Input: part model. Units: mm. Frame: model coordinates. A direction names the side the tool comes from. Coordinates: 2 decimals unless noted, no trailing zeros. Order: outer loops, then holes, each group sorted by start corner. A loop starts at its lowest first (then second) coordinate and runs counter-clockwise, first axis right, second up. Notation, with made-up numbers: (-0.5, -8.5) - (50.5, -8.5) arc R31 cw to (50.5, 26.5) - close; hole circle Ø2 at (18, 39.25). An arc over 180 degrees is marked (long way). Answer as CSV lines item,"result". Start each with the question number.
Item 1: Section A-A (x = 0). Output: boundary loops of the cut face in (y, z) (3 decimals), and give its area (3 significant figures).
Item 2: Material intervals for line 1 along Y through (x, z) = (0, 22.55) (3 decimals); line 2 along X through (y, z) = (10.25, 22); line 3 along Z through (x, y) = (-28, 3.25), sorted ascending.
Item 3: Section B-B (y = 13.5). Output: boundary loops of the cut face in (x, z).
Item 4: Section D-D (z = -11.5). Output: boundary loops of the cut face in (x, y), and give its area (3 significant figures).
Item 5: Section C-C (x = 7). Output: boundary loops of the cut face in (y, z).
Item 6: First-contact query: pin 1 (3.5 mm diameter, centred on x = 0, y = 7.5, fed in from +Z); pin 2 (6 mm diameter, centred on x = -24, z = -12.5, fed in from -Y); pin 3 (7.5 mm diameter, centred on y = 9.5, z = -7, fed in from -X); pin 4 (8 mm diameter, centred on y = 7, z = 9, fed in from -X). Flat tips, straight axial feed; report the tip coordinate or a pass-through.
Item 7: Draft query along X for faces 4 (the flat face through (22, 8, 1)), 5 (the cylindrical face through (-26.537, 6.686, 22.535)), 6 (the flat face through (-32.2, 7.4, 17)). Return one class per face: +X half, -X half, draft (parallel to the pull), parting line (faces both ways), or undercut.
Item 8: Access query for faces 1 (the flat face through (0, 4, 18)), 2 (the flat face through (-26.9, 5.8, 20)), 3 (the flat face through (-1, 0, 17)). Directions: +Z, -Z, +X, -X, +Y, -Y. A direction counts if a zero-diameter tool reaches every point of the face in a straight line with its end or side. Return the directions, or none.
from build123d import *

# Parameters (mm, degrees)
CROQUIS1_R              = 15
SALIENTE_EXTRUIR1_DEPTH = 15
CORTAR_EXTRUIR1_REACH   = 62.49
CROQUIS2_R              = 2.125
CORTAR_EXTRUIR2_DEPTH   = 3
CUT_EXTRUDE1_DEPTH      = 46.552167984
CUT_EXTRUDE2_REACH      = 66.49
CUT_EXTRUDE2_END_RADIUS = 15
CUT_EXTRUDE2_START      = -4
CUT_EXTRUDE3_START      = -39
CUT_EXTRUDE3_DEPTH      = 3
BOSS_EXTRUDE3_START     = -15
BOSS_EXTRUDE3_DEPTH     = 15
CUT_EXTRUDE4_START      = -20
SKETCH4_R               = 1.625
CUT_EXTRUDE4_DEPTH      = 41.489668539


with BuildPart() as part:
    # Croquis1 → Saliente-Extruir1 (new body)
    with BuildSketch(Plane(origin=(0, 0, 0), x_dir=(1, 0, 0), z_dir=(0, 1, 0))):
        with BuildLine():
            Line((-35, -17), (-35, -25))
            Line((-35, -25), (35, -25))
            Line((35, -25), (35, -17))
            Line((35, -17), (25, -17))
            Line((25, -17), (22, 0))
            ThreePointArc((22, 0), (0, 22), (-22, 0))
            Line((-22, 0), (-25, -17))
            Line((-25, -17), (-35, -17))
        make_face()
        with Locations(Location((0, 0, 0), (0, 0, 270))):
            Circle(CROQUIS1_R, mode=Mode.SUBTRACT)
    extrude(amount=SALIENTE_EXTRUIR1_DEPTH)

    # Croquis2 → Cortar-Extruir1 (cut, up to next)
    with BuildSketch(Plane.XY.offset(25), mode=Mode.PRIVATE) as cortar_extruir1_sk1:
        with Locations((-28.5, 7.5)):
            Circle(CROQUIS2_R)
    cortar_extruir1_tool1 = extrude(cortar_extruir1_sk1.sketch, amount=-CORTAR_EXTRUIR1_REACH, mode=Mode.PRIVATE) & part.part
    # Croquis2 → Cortar-Extruir1 (cut, up to next)
    with BuildSketch(Plane.XY.offset(25), mode=Mode.PRIVATE) as cortar_extruir1_sk2:
        with Locations((28.5, 7.5)):
            Circle(CROQUIS2_R)
    cortar_extruir1_tool2 = extrude(cortar_extruir1_sk2.sketch, amount=-CORTAR_EXTRUIR1_REACH, mode=Mode.PRIVATE) & part.part
    # Croquis2 → Cortar-Extruir1 (cut, up to next)
    with BuildSketch(Plane.XY.offset(25), mode=Mode.PRIVATE) as cortar_extruir1_sk3:
        with Locations((0, 7.5)):
            Circle(CROQUIS2_R)
    cortar_extruir1_tool3 = extrude(cortar_extruir1_sk3.sketch, amount=-CORTAR_EXTRUIR1_REACH, mode=Mode.PRIVATE) & part.part
    add(cortar_extruir1_tool1.solids().sort_by_distance((-28.5, 7.5, 25))[0], mode=Mode.SUBTRACT)
    add(cortar_extruir1_tool2.solids().sort_by_distance((28.5, 7.5, 25))[0], mode=Mode.SUBTRACT)
    add(cortar_extruir1_tool3.solids().sort_by_distance((0, 7.5, 25))[0], mode=Mode.SUBTRACT)

    # Croquis3 → Cortar-Extruir2 (cut)
    with BuildSketch(Plane(origin=(0, 0, 17), x_dir=(-1, 0, 0), z_dir=(0, 0, -1))):
        Polygon((25, 5.479274058), (28.5, 3.458548116), (32, 5.479274058), (32, 9.520725942), (28.5, 11.541451884), (25, 9.520725942), align=None)
        Polygon((-25, 5.479274058), (-25, 9.520725942), (-28.5, 11.541451884), (-32, 9.520725942), (-32, 5.479274058), (-28.5, 3.458548116), align=None)
    extrude(amount=-CORTAR_EXTRUIR2_DEPTH, mode=Mode.SUBTRACT)

    # Sketch1 → Cut-Extrude1 (cut, through all)
    with BuildSketch(Plane(origin=(0, 15, 0), x_dir=(1, 0, 0), z_dir=(0, 1, 0))):
        Polygon((22, -25), (22, -20), (17, -25), align=None)
        Polygon((22, 0), (22, -20), (22, -25), (35, -25), (35, -17), (25, -17), align=None)
    extrude(amount=-CUT_EXTRUDE1_DEPTH, mode=Mode.SUBTRACT)

    # Cut-Extrude2: up to this cylinder (the profile starts outside it)
    cut_extrude2_end = Plane(origin=(0, 7.5, 0), z_dir=(0, -1, 0)) * Cylinder(CUT_EXTRUDE2_END_RADIUS, 163.98, mode=Mode.PRIVATE)
    # Sketch2 → Cut-Extrude2 (cut, up to the surface)
    with BuildSketch(Plane.XY.offset(25).offset(CUT_EXTRUDE2_START), mode=Mode.PRIVATE) as cut_extrude2_sk1:
        Polygon((2.020725942, 4), (4.041451884, 7.5), (2.020725942, 11), (-2.020725942, 11), (-4.041451884, 7.5), (-2.020725942, 4), align=None)
    cut_extrude2_tool1 = extrude(cut_extrude2_sk1.sketch, amount=-CUT_EXTRUDE2_REACH, mode=Mode.PRIVATE) - cut_extrude2_end
    add(cut_extrude2_tool1.solids().sort_by_distance((0, 7.5, 21))[0], mode=Mode.SUBTRACT)

    # Sketch3 → Cut-Extrude3 (cut)
    with BuildSketch(Plane.XY.offset(25).offset(CUT_EXTRUDE3_START)):
        Polygon((1.58771324, 4.75), (3.175426481, 7.5), (1.58771324, 10.25), (-1.58771324, 10.25), (-3.175426481, 7.5), (-1.58771324, 4.75), align=None)
    extrude(amount=-CUT_EXTRUDE3_DEPTH, mode=Mode.SUBTRACT)

    # Sketch5 → Boss-Extrude3 (add)
    with BuildSketch(Plane(origin=(0, 15, 0), x_dir=(1, 0, 0), z_dir=(0, 1, 0)).offset(BOSS_EXTRUDE3_START)):
        with BuildLine():
            ThreePointArc((-12.177948568, 18.322051432), (-6.36061571, 21.060450323), (3.35e-07, 22))
            Line((3.35e-07, 22), (-17, 22))
            ThreePointArc((-17, 22), (-13.967695362, 20.975566448), (-12.177948568, 18.322051432))
        make_face()
        with BuildLine():
            ThreePointArc((12.177948568, 18.322051432), (13.967695362, 20.975566448), (17, 22))
            Line((17, 22), (3.35e-07, 22))
            ThreePointArc((3.35e-07, 22), (6.360616031, 21.060450226), (12.177948568, 18.322051432))
        make_face()
        with BuildLine():
            ThreePointArc((18.322051432, 12.177948568), (20.975566448, 13.967695362), (22, 17))
            ThreePointArc((22, 17), (20.535533906, 20.535533906), (17, 22))
            ThreePointArc((17, 22), (13.967695362, 20.975566448), (12.177948568, 18.322051432))
            ThreePointArc((12.177948568, 18.322051432), (15.556349186, 15.556349186), (18.322051432, 12.177948568))
        make_face()
        with BuildLine():
            ThreePointArc((12.177948568, 18.322051432), (13.464466094, 13.464466094), (18.322051432, 12.177948568))
            ThreePointArc((18.322051432, 12.177948568), (15.556349186, 15.556349186), (12.177948568, 18.322051432))
        make_face()
        with BuildLine():
            ThreePointArc((18.322051432, 12.177948568), (21.060450274, 6.36061587), (22, 0))
            Line((22, 0), (22, 17))
            ThreePointArc((22, 17), (20.975566448, 13.967695362), (18.322051432, 12.177948568))
        make_face()
        with BuildLine():
            ThreePointArc((-17, 22), (-20.535533906, 20.535533906), (-22, 17))
            ThreePointArc((-22, 17), (-20.975566448, 13.967695362), (-18.322051432, 12.177948568))
            ThreePointArc((-18.322051432, 12.177948568), (-15.556349186, 15.556349186), (-12.177948568, 18.322051432))
            ThreePointArc((-12.177948568, 18.322051432), (-13.967695362, 20.975566448), (-17, 22))
        make_face()
        with BuildLine():
            ThreePointArc((-12.177948568, 18.322051432), (-15.556349186, 15.556349186), (-18.322051432, 12.177948568))
            ThreePointArc((-18.322051432, 12.177948568), (-13.967695362, 13.024433552), (-12, 17))
            ThreePointArc((-12, 17), (-12.044686833, 17.666986822), (-12.177948568, 18.322051432))
        make_face()
        with BuildLine():
            Line((-22, 17), (-22, 0))
            ThreePointArc((-22, 0), (-21.060450274, 6.36061587), (-18.322051432, 12.177948568))
            ThreePointArc((-18.322051432, 12.177948568), (-20.975566448, 13.967695362), (-22, 17))
        make_face()
    extrude(amount=BOSS_EXTRUDE3_DEPTH)

    # Sketch4 → Cut-Extrude4 (cut, through all)
    with BuildSketch(Plane.XY.offset(25).offset(CUT_EXTRUDE4_START)):
        with Locations((0, 7.5)):
            Circle(SKETCH4_R)
    extrude(amount=-CUT_EXTRUDE4_DEPTH, mode=Mode.SUBTRACT)


solid = part.part
Determined:
1,outline,"(0, -22) - (5.875, -22) - (5.875, -17) - (4.75, -17) - (4.75, -15) - (0, -15) - close; (0, 15) - (4, 15) - (4, 21) - (5.375, 21) - (5.375, 25) - (0, 25) - close; (9.125, -22) - (15, -22) - (15, -15) - (10.25, -15) - (10.25, -17) - (9.125, -17) - close; (9.625, 21) - (11, 21) - (11, 15) - (15, 15) - (15, 25) - (9.625, 25) - close"
1,area,"169 mm^2"
2,line 1,"y = 0 to 5.375, 9.625 to 15"
2,line 2,"x = -35 to 20"
2,line 3,"z = 17 to 25"
3,outline,"(-35, 17) - (-25, 17) - (-22, 0) - (-22, -17) arc R5 ccw to (-17, -22) - (17, -22) arc R5 ccw to (22, -17) - (22, 20) - (17, 25) - (-35, 25) - close; hole circle Ø30 at (0, 0)"
4,outline,"(-22, 0) - (-9.63, 0) - (-9.63, 15) - (-22, 15) - close; (9.63, 0) - (22, 0) - (22, 15) - (9.63, 15) - close"
4,area,"371 mm^2"
5,outline,"(0, -22) - (15, -22) - (15, -13.27) - (0, -13.27) - close; (0, 13.27) - (15, 13.27) - (15, 25) - (0, 25) - close"
6,pin 1,"stops at z = -17"
6,pin 2,"stops at y = 0"
6,pin 3,"stops at x = -22"
6,pin 4,"stops at x = -24.29"
7,face 4,"+X half"
7,face 5,"undercut"
7,face 6,"draft"
8,face 1,"none"
8,face 2,"-Z"
8,face 3,"+Z, -Z, +X, -X, -Y"
